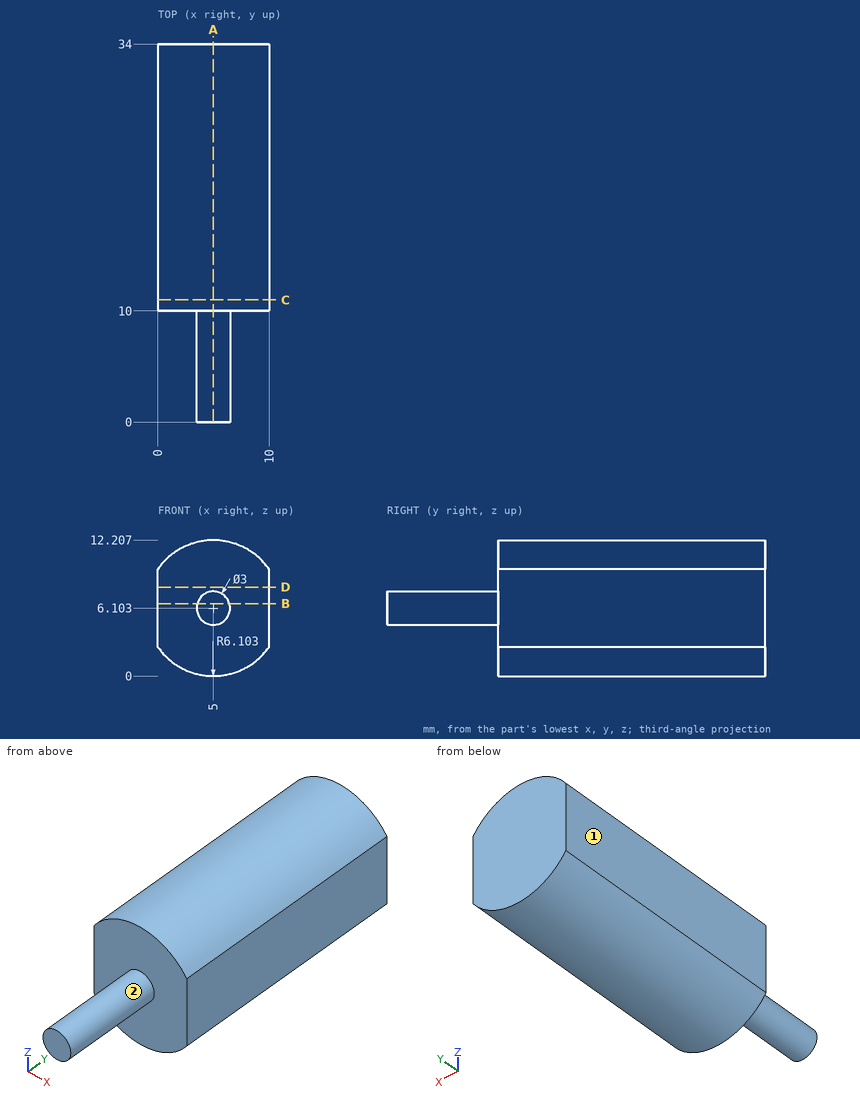
The figure shows three views and two pictorial views of one solid part (mm, origin at its lowest corner). Answer the questions. A direction names the side the tool comes from. Give positions to 0.01 mm unless a question says otherwise; leave off trailing zeros. Write each loop counter-clockwise with the first axis right and the second up, starting at its lowest first coordinate (ties: lowest second). Pieces come first, ordered by that corner, then holes. Notation, with made-up numbers: (77, -22) -> (105, -22) arc R13 cw to (105, -15) -> close; hole circle Ø4 at (29, 76). An arc over 180 degrees is marked (long way). Use one line per item in the form item = value.
1) Section D-D on z = 8 is taken. Write down the section's boundary in (x, y).
Result:
outline = (0, 10) -> (10, 10) -> (10, 34) -> (0, 34) -> close
2) Section C-C on y = 11 is taken. Write down the section's boundary in (x, z).
Result:
outline = (0, 2.6) arc R6.1 ccw to (10, 2.6) -> (10, 9.6) arc R6.1 ccw to (0, 9.6) -> close
3) Each of these flat-tipped pins is pushed along its axis until it touches: P1, Ø3, axis at x = 8, y = 25, coming from the +Z side; P2, Ø3, axis at x = 8.5, z = 7, coming from the -Y side; P3, Ø2, axis at x = 2, y = 27.5, coming from the +Z side. Where does it stop, or does it pass through?
Result:
P1 = 12.02
P2 = 10
P3 = 11.87
4) A tool of negligible diameter and unlimited length cuts with its end or side. For the marked faces 1 and 2, from which of +Z, -Z, +X, -X, +Y, -Y can it reach the whole face along a straight path? Write none if from no direction.
Result:
face_1 = +Z, -Z, -X, +Y, -Y
face_2 = -Y
5) Straight lines are drawn through the part: probe 1 along Y at (x, z) = (6.25, 9.75); probe 2 along X at (y, z) = (7, 6.25); probe 3 along Z at (x, y) = (1.5, 28) (1 decimal). For each, find the intervals that lie inside material, in ascending order.
Result:
probe_1 = 10 to 34
probe_2 = 3.51 to 6.49
probe_3 = 1.1 to 11.1
6) Section B-B on z = 6.5 is taken. Write down the section's boundary in (x, y), plus the area to 3 significant figures.
Result:
outline = (0, 10) -> (3.55, 10) -> (3.55, 0) -> (6.45, 0) -> (6.45, 10) -> (10, 10) -> (10, 34) -> (0, 34) -> close
area = 269 mm²
7) Section A-A on x = 5 is taken. Write down the section's boundary in (y, z), plus the area to 3 significant figures.
Result:
outline = (0, 4.6) -> (10, 4.6) -> (10, 0) -> (34, 0) -> (34, 12.21) -> (10, 12.21) -> (10, 7.6) -> (0, 7.6) -> close
area = 323 mm²
